```python
from build123d import *
from build123d.topology import SkipClean

# Parameters (mm, degrees)
SKETCH2_R           = 6.575
BOSS_EXTRUDE1_DEPTH = 5
SKETCH3_R           = 4.5
BOSS_EXTRUDE2_DEPTH = 10
SKETCH4_R           = 2.125
BOSS_EXTRUDE3_DEPTH = 4
SKETCH5_R           = 1.8
BOSS_EXTRUDE4_DEPTH = 3
BOSS_EXTRUDE5_DEPTH = 10
CUT_EXTRUDE1_START  = -10
CUT_EXTRUDE1_DEPTH  = 10
SKETCH8_R           = 3.075
BOSS_EXTRUDE6_DEPTH = 12
CUT_EXTRUDE2_DEPTH  = 10


with BuildPart() as part:
    # Sketch2 → Boss-Extrude1 (new body)
    with BuildSketch(Plane.XY):
        with BuildLine():
            Line((-20, 0), (-20, -97))
            ThreePointArc((-20, -97), (0, -117), (20, -97))
            Line((20, -97), (20, 0))
            ThreePointArc((20, 0), (0, 20), (-20, 0))
        make_face()
        Circle(SKETCH2_R, mode=Mode.SUBTRACT)
    extrude(amount=BOSS_EXTRUDE1_DEPTH)

    # Sketch3 → Boss-Extrude2 (add)
    with BuildSketch(Plane.XY.offset(5)):
        with Locations((0, -97)):
            Circle(SKETCH3_R)
    extrude(amount=BOSS_EXTRUDE2_DEPTH)

    # Sketch4 → Boss-Extrude3 (add)
    with BuildSketch(Plane.XY.offset(5)):
        with Locations((-8, 8)):
            Circle(SKETCH4_R)
        with Locations((8, 8)):
            Circle(SKETCH4_R)
        with Locations((8, -8)):
            Circle(SKETCH4_R)
        with Locations((-8, -8)):
            Circle(SKETCH4_R)
    extrude(amount=BOSS_EXTRUDE3_DEPTH)

    # Sketch5 → Boss-Extrude4 (add)
    with BuildSketch(Plane.XY.offset(9)):
        with Locations((-8, 8)):
            Circle(SKETCH5_R)
        with Locations((8, 8)):
            Circle(SKETCH5_R)
        with Locations((8, -8)):
            Circle(SKETCH5_R)
        with Locations((-8, -8)):
            Circle(SKETCH5_R)
    extrude(amount=BOSS_EXTRUDE4_DEPTH)

    # Sketch6 → Boss-Extrude5 (add)
    with BuildSketch(Plane.XY.offset(5)):
        with BuildLine():
            Line((20, -97), (20, 0))
            ThreePointArc((20, 0), (0, 20), (-20, 0))
            Line((-20, 0), (-20, -97))
            ThreePointArc((-20, -97), (0, -117), (20, -97))
        make_face()
        with BuildLine():
            Line((-19, 0), (-19, -97))
            ThreePointArc((-19, -97), (0, -116), (19, -97))
            Line((19, -97), (19, 0))
            ThreePointArc((19, 0), (0, 19), (-19, 0))
        make_face(mode=Mode.SUBTRACT)
    extrude(amount=BOSS_EXTRUDE5_DEPTH)

    # Sketch7 → Cut-Extrude1 (cut)
    with BuildSketch(Plane.XY.offset(5).offset(CUT_EXTRUDE1_START)):
        with BuildLine():
            Line((-10.125, 8), (-10.125, -8))
            ThreePointArc((-10.125, -8), (-9.50260191, -6.49739809), (-8, -5.875))
            Line((-8, -5.875), (-8, 5.875))
            ThreePointArc((-8, 5.875), (-9.50260191, 6.49739809), (-10.125, 8))
        make_face()
        with BuildLine():
            Line((-8, -10.125), (8, -10.125))
            ThreePointArc((8, -10.125), (6.49739809, -9.50260191), (5.875, -8))
            Line((5.875, -8), (-5.875, -8))
            ThreePointArc((-5.875, -8), (-6.49739809, -9.50260191), (-8, -10.125))
        make_face()
        with BuildLine():
            Line((10.125, -8), (10.125, 8))
            ThreePointArc((10.125, 8), (9.50260191, 6.49739809), (8, 5.875))
            Line((8, 5.875), (8, -5.875))
            ThreePointArc((8, -5.875), (9.50260191, -6.49739809), (10.125, -8))
        make_face()
        with BuildLine():
            Line((8, 10.125), (-8, 10.125))
            ThreePointArc((-8, 10.125), (-6.49739809, 9.50260191), (-5.875, 8))
            Line((-5.875, 8), (5.875, 8))
            ThreePointArc((5.875, 8), (6.49739809, 9.50260191), (8, 10.125))
        make_face()
    extrude(amount=CUT_EXTRUDE1_DEPTH, mode=Mode.SUBTRACT)

    # Sketch8 → Boss-Extrude6 (add)
    with BuildSketch(Plane.XY.offset(15)):
        with Locations((0, -97)):
            Circle(SKETCH8_R)
    extrude(amount=BOSS_EXTRUDE6_DEPTH)

    # Sketch10 → Cut-Extrude2 (cut)
    with SkipClean():  # the faces are left unmerged after this step: merging them gives an invalid solid
        with BuildSketch(Plane(origin=(0, 0, 0), x_dir=(-1, 0, 0), z_dir=(0, 0, -1))):
            with BuildLine():
                Line((-8, 10.125), (-11.181980515, 13.306980515))
                ThreePointArc((-11.181980515, 13.306980515), (0, 17.938708499), (11.181980515, 13.306980515))
                Line((11.181980515, 13.306980515), (8, 10.125))
                Line((8, 10.125), (-8, 10.125))
            make_face()
            with BuildLine():
                Line((-10.125, 8), (-13.306980515, 11.181980515))
                ThreePointArc((-13.306980515, 11.181980515), (-17.938708499, 0), (-13.306980515, -11.181980515))
                Line((-13.306980515, -11.181980515), (-10.125, -8))
                Line((-10.125, -8), (-10.125, 8))
            make_face()
            with BuildLine():
                Line((10.125, 8), (13.306980515, 11.181980515))
                ThreePointArc((13.306980515, 11.181980515), (17.938708499, 0), (13.306980515, -11.181980515))
                Line((13.306980515, -11.181980515), (10.125, -8))
                Line((10.125, -8), (10.125, 8))
            make_face()
            with BuildLine():
                Line((8, -10.125), (11.181980515, -13.306980515))
                ThreePointArc((11.181980515, -13.306980515), (0, -17.938708499), (-11.181980515, -13.306980515))
                Line((-11.181980515, -13.306980515), (-8, -10.125))
                Line((-8, -10.125), (8, -10.125))
            make_face()
        extrude(amount=-CUT_EXTRUDE2_DEPTH, mode=Mode.SUBTRACT)


solid = part.part
```
The model under review builds one solid part; all positions refer to its coordinate system, in mm. A direction names the side the tool comes from. Give positions to 0.01 mm unless a question says otherwise; leave off trailing zeros. Write each loop counter-clockwise with the first axis right and the second up, starting at its lowest first coordinate (ties: lowest second). Pieces come first, ordered by that corner, then holes. Notation, with made-up numbers: M -30.75,85 L -23.75,85 A27 ccw -23.75,105 Z; hole C -37.75,-2 d2. An arc over 180 degrees is marked long. Write item = value, one per line. Start each with the question number.
Q1. Clearance check with flat-ended pins moving along their axes: pin 1 (10 mm diameter, centred on x = 7, z = 14, fed in from -Y); pin 2 (12 mm diameter, centred on x = -7, y = -42.5, fed in from +Z); pin 3 (8 mm diameter, centred on y = -60, z = 17, fed in from +X); pin 4 (12 mm diameter, centred on x = 12.5, z = 18, fed in from +Y). State where each tip first meets the part, or that it passes through.
Q2. We need section A-A (z = 10.5). State the section outline as (x, y) points.
Q3. Machinability: for faces 4 (the face through (8, 0, 2)), 5 (the face through (7, 0, 5)), which of the approach directions +Z, -Z, +X, -X, +Y, -Y give a long, thin tool a straight path to every point of the face, cutting with its end or side? Answer none if there is none.
Q4. We need section C-C (z = 18). State the section outline as (x, y) points (3 decimals), plus the area to 3 significant figures.
Q5. Mouldability with a two-part tool opening along X and no side actions: class faces 1 (the face through (20, -49, 7)), 2 (the face through (-9.613, 11.738, 2.465)), 3 (the face through (0, 20, 7)) as released by +X, released by -X, zero draft, split by the parting line, or undercut.
Q6. For line 1 (Y direction, x = 0, z = 3.8) (3 decimals); line 2 (X direction, y = -71, z = 5.5); line 3 (X direction, y = -1, z = 3.75), list the stretches that pass through material, from the lowest coordinate up.
Q7. We need section B-B (y = -38). State the section outline as (x, z) points.
Result set:
q1.pin_1 = -116.9
q1.pin_2 = 5
q1.pin_3 = 20
q1.pin_4 = 18.62
q2.outline = M -20,-97 A20 ccw 20,-97 L 20,0 A20 ccw -20,0 Z; C -8,-8 d3.6; C -8,8 d3.6; C 0,-97 d9; C 8,-8 d3.6; C 8,8 d3.6; hole M -19,-97 A19 ccw 19,-97 L 19,0 A19 ccw -19,0 Z
q3.face_4 = +Z, -Z
q3.face_5 = +Z
q4.outline = C 0,-97 d6.15
q4.area = 29.7 mm2
q5.face_1 = released by +X
q5.face_2 = undercut
q5.face_3 = split by the parting line
q6.line_1 = -117 to -17.939, -8 to -6.575, 6.575 to 8, 17.939 to 20
q6.line_2 = -20 to -19, 19 to 20
q6.line_3 = -20 to -17.91, -8 to -6.5, 6.5 to 8, 17.91 to 20
q7.outline = M -20,0 L 20,0 L 20,15 L 19,15 L 19,5 L -19,5 L -19,15 L -20,15 Z
